Read the model definition and answer for the solid it produces. Units are mm, in the model's axes. Coordinates: 2 decimals unless noted, no trailing zeros.
(1) Straight lines are drawn through the part: line 1 along X through (y, z) = (291.5, -4.5); line 2 along Z through (x, y) = (8.5, 274.5); line 3 along Z through (x, y) = (-12, 164.5). For each, find the intervals that lie inside material, in ascending order.
(2) The part is cut by section A-A, the plane y = 192. State how many separate pieces and enclosed holes the cut face has, and give its area (3 significant figures).
(3) Given pin 1 (1.2 mm diameter, centred on x = -25, y = 241.5, fed in from +Z); pin 2 (0.6 mm diameter, centred on y = 140.5, z = 14.5, fed in from -X); pin 3 (1.3 mm diameter, centred on y = 270, z = 28.5, fed in from +X), each flat-ended and moving along its own axis, determine where each tip first touches the part or whether it passes through.
```python
from build123d import *

# Parameters (mm, degrees)
BOSS_EXTRUDE1_DEPTH = 500


with BuildPart() as part:
    # Sketch1 → Boss-Extrude1 (new body)
    with BuildSketch(Plane(origin=(0, 0, 0), x_dir=(1, 0, 0), z_dir=(0, 1, 0))):
        with BuildLine():
            Line((-27.932618907, -6.859852703), (-27.932618907, 5.140147297))
            ThreePointArc((-27.932618907, 5.140147297), (-26.761046031, 7.968574422), (-23.932618907, 9.140147297))
            Line((-23.932618907, 9.140147297), (-11.932618907, 9.140147297))
            Line((-11.932618907, 9.140147297), (-11.932618907, 4.640147297))
            Line((-11.932618907, 4.640147297), (-19.182618907, 4.640147297))
            Line((-19.182618907, 4.640147297), (-19.182618907, 3.140147297))
            Line((-19.182618907, 3.140147297), (-12.932618907, -3.109852703))
            Line((-12.932618907, -3.109852703), (-7.932618907, -3.109852703))
            Line((-7.932618907, -3.109852703), (-2.932618907, -3.109852703))
            Line((-2.932618907, -3.109852703), (3.317381093, 3.140147297))
            Line((3.317381093, 3.140147297), (3.317381093, 4.640147297))
            Line((3.317381093, 4.640147297), (-3.932618907, 4.640147297))
            Line((-3.932618907, 4.640147297), (-3.932618907, 9.140147297))
            Line((-3.932618907, 9.140147297), (8.067381093, 9.140147297))
            ThreePointArc((8.067381093, 9.140147297), (10.895808218, 7.968574422), (12.067381093, 5.140147297))
            Line((12.067381093, 5.140147297), (12.067381093, -6.859852703))
            Line((12.067381093, -6.859852703), (7.567381093, -6.859852703))
            Line((7.567381093, -6.859852703), (7.567381093, 0.390147297))
            Line((7.567381093, 0.390147297), (6.067381093, 0.390147297))
            Line((6.067381093, 0.390147297), (-0.182618907, -5.859852703))
            Line((-0.182618907, -5.859852703), (-0.182618907, -10.859852703))
            Line((-0.182618907, -10.859852703), (-0.182618907, -15.859852703))
            Line((-0.182618907, -15.859852703), (6.067381093, -22.109852703))
            Line((6.067381093, -22.109852703), (7.567381093, -22.109852703))
            Line((7.567381093, -22.109852703), (7.567381093, -14.859852703))
            Line((7.567381093, -14.859852703), (12.067381093, -14.859852703))
            Line((12.067381093, -14.859852703), (12.067381093, -26.859852703))
            ThreePointArc((12.067381093, -26.859852703), (10.895808218, -29.688279827), (8.067381093, -30.859852703))
            Line((8.067381093, -30.859852703), (-3.932618907, -30.859852703))
            Line((-3.932618907, -30.859852703), (-3.932618907, -26.359852703))
            Line((-3.932618907, -26.359852703), (3.317381093, -26.359852703))
            Line((3.317381093, -26.359852703), (3.317381093, -24.859852703))
            Line((3.317381093, -24.859852703), (-2.932618907, -18.609852703))
            Line((-2.932618907, -18.609852703), (-7.932618907, -18.609852703))
            Line((-7.932618907, -18.609852703), (-12.932618907, -18.609852703))
            Line((-12.932618907, -18.609852703), (-19.182618907, -24.859852703))
            Line((-19.182618907, -24.859852703), (-19.182618907, -26.359852703))
            Line((-19.182618907, -26.359852703), (-11.932618907, -26.359852703))
            Line((-11.932618907, -26.359852703), (-11.932618907, -30.859852703))
            Line((-11.932618907, -30.859852703), (-23.932618907, -30.859852703))
            ThreePointArc((-23.932618907, -30.859852703), (-26.761046031, -29.688279827), (-27.932618907, -26.859852703))
            Line((-27.932618907, -26.859852703), (-27.932618907, -14.859852703))
            Line((-27.932618907, -14.859852703), (-23.432618907, -14.859852703))
            Line((-23.432618907, -14.859852703), (-23.432618907, -22.109852703))
            Line((-23.432618907, -22.109852703), (-21.932618907, -22.109852703))
            Line((-21.932618907, -22.109852703), (-15.682618907, -15.859852703))
            Line((-15.682618907, -15.859852703), (-15.682618907, -10.859852703))
            Line((-15.682618907, -10.859852703), (-15.682618907, -5.859852703))
            Line((-15.682618907, -5.859852703), (-21.932618907, 0.390147297))
            Line((-21.932618907, 0.390147297), (-23.432618907, 0.390147297))
            Line((-23.432618907, 0.390147297), (-23.432618907, -6.859852703))
            Line((-23.432618907, -6.859852703), (-27.932618907, -6.859852703))
        make_face()
        with BuildLine():
            Line((-25.932618907, 2.390147297), (-25.932618907, 5.140147297))
            ThreePointArc((-25.932618907, 5.140147297), (-25.346832469, 6.55436086), (-23.932618907, 7.140147297))
            Line((-23.932618907, 7.140147297), (-21.182618907, 7.140147297))
            Line((-21.182618907, 7.140147297), (-21.182618907, 3.097254079))
            Line((-21.182618907, 3.097254079), (-20.734395602, 2.649030774))
            Line((-20.734395602, 2.649030774), (-21.441502383, 1.941923993))
            Line((-21.441502383, 1.941923993), (-21.889725688, 2.390147297))
            Line((-21.889725688, 2.390147297), (-25.932618907, 2.390147297))
        make_face(mode=Mode.SUBTRACT)
        with BuildLine():
            Line((-20.380842211, 0.881263821), (-13.682618907, -5.816959484))
            Line((-13.682618907, -5.816959484), (-13.682618907, -7.955115193))
            Line((-13.682618907, -7.955115193), (-13.182618907, -7.955115193))
            Line((-13.182618907, -7.955115193), (-12.002324056, -7.955115193))
            ThreePointArc((-12.002324056, -7.955115193), (-11.468152813, -7.324318797), (-10.837356416, -6.790147554))
            Line((-10.837356416, -6.790147554), (-10.837356416, -5.609852703))
            Line((-10.837356416, -5.609852703), (-10.837356416, -5.109852703))
            Line((-10.837356416, -5.109852703), (-12.975512126, -5.109852703))
            Line((-12.975512126, -5.109852703), (-19.67373543, 1.588370602))
            Line((-19.67373543, 1.588370602), (-20.380842211, 0.881263821))
        make_face(mode=Mode.SUBTRACT)
        with BuildLine():
            Line((10.067381093, 2.390147297), (10.067381093, 5.140147297))
            ThreePointArc((10.067381093, 5.140147297), (9.481594656, 6.55436086), (8.067381093, 7.140147297))
            Line((8.067381093, 7.140147297), (5.317381093, 7.140147297))
            Line((5.317381093, 7.140147297), (5.317381093, 3.097254079))
            Line((5.317381093, 3.097254079), (4.869157789, 2.649030774))
            Line((4.869157789, 2.649030774), (5.57626457, 1.941923993))
            Line((5.57626457, 1.941923993), (6.024487874, 2.390147297))
            Line((6.024487874, 2.390147297), (10.067381093, 2.390147297))
        make_face(mode=Mode.SUBTRACT)
        with BuildLine():
            Line((-2.182618907, -5.816959484), (-2.182618907, -7.955115193))
            Line((-2.182618907, -7.955115193), (-2.682618907, -7.955115193))
            Line((-2.682618907, -7.955115193), (-3.862913758, -7.955115193))
            ThreePointArc((-3.862913758, -7.955115193), (-4.397085001, -7.324318797), (-5.027881397, -6.790147554))
            Line((-5.027881397, -6.790147554), (-5.027881397, -5.609852703))
            Line((-5.027881397, -5.609852703), (-5.027881397, -5.109852703))
            Line((-5.027881397, -5.109852703), (-2.889725688, -5.109852703))
            Line((-2.889725688, -5.109852703), (3.808497617, 1.588370602))
            Line((3.808497617, 1.588370602), (4.515604398, 0.881263821))
            Line((4.515604398, 0.881263821), (-2.182618907, -5.816959484))
        make_face(mode=Mode.SUBTRACT)
        with BuildLine():
            Line((5.317381093, -28.859852703), (8.067381093, -28.859852703))
            ThreePointArc((8.067381093, -28.859852703), (9.481594656, -28.274066265), (10.067381093, -26.859852703))
            Line((10.067381093, -26.859852703), (10.067381093, -24.109852703))
            Line((10.067381093, -24.109852703), (6.024487874, -24.109852703))
            Line((6.024487874, -24.109852703), (5.57626457, -23.661629398))
            Line((5.57626457, -23.661629398), (4.869157789, -24.368736179))
            Line((4.869157789, -24.368736179), (5.317381093, -24.816959484))
            Line((5.317381093, -24.816959484), (5.317381093, -28.859852703))
        make_face(mode=Mode.SUBTRACT)
        with BuildLine():
            Line((-2.889725688, -16.609852703), (-5.027881397, -16.609852703))
            Line((-5.027881397, -16.609852703), (-5.027881397, -16.109852703))
            Line((-5.027881397, -16.109852703), (-5.027881397, -14.929557852))
            ThreePointArc((-5.027881397, -14.929557852), (-4.397085001, -14.395386609), (-3.862913758, -13.764590212))
            Line((-3.862913758, -13.764590212), (-2.682618907, -13.764590212))
            Line((-2.682618907, -13.764590212), (-2.182618907, -13.764590212))
            Line((-2.182618907, -13.764590212), (-2.182618907, -15.902745921))
            Line((-2.182618907, -15.902745921), (4.515604398, -22.600969226))
            Line((4.515604398, -22.600969226), (3.808497617, -23.308076007))
            Line((3.808497617, -23.308076007), (-2.889725688, -16.609852703))
        make_face(mode=Mode.SUBTRACT)
        with BuildLine():
            Line((-25.932618907, -24.109852703), (-25.932618907, -26.859852703))
            ThreePointArc((-25.932618907, -26.859852703), (-25.346832469, -28.274066265), (-23.932618907, -28.859852703))
            Line((-23.932618907, -28.859852703), (-21.182618907, -28.859852703))
            Line((-21.182618907, -28.859852703), (-21.182618907, -24.816959484))
            Line((-21.182618907, -24.816959484), (-20.734395602, -24.368736179))
            Line((-20.734395602, -24.368736179), (-21.441502383, -23.661629398))
            Line((-21.441502383, -23.661629398), (-21.889725688, -24.109852703))
            Line((-21.889725688, -24.109852703), (-25.932618907, -24.109852703))
        make_face(mode=Mode.SUBTRACT)
        with BuildLine():
            Line((-13.682618907, -15.902745921), (-13.682618907, -13.764590212))
            Line((-13.682618907, -13.764590212), (-13.182618907, -13.764590212))
            Line((-13.182618907, -13.764590212), (-12.002324056, -13.764590212))
            ThreePointArc((-12.002324056, -13.764590212), (-11.468152813, -14.395386609), (-10.837356416, -14.929557852))
            Line((-10.837356416, -14.929557852), (-10.837356416, -16.109852703))
            Line((-10.837356416, -16.109852703), (-10.837356416, -16.609852703))
            Line((-10.837356416, -16.609852703), (-12.975512126, -16.609852703))
            Line((-12.975512126, -16.609852703), (-19.67373543, -23.308076007))
            Line((-19.67373543, -23.308076007), (-20.380842211, -22.600969226))
            Line((-20.380842211, -22.600969226), (-13.682618907, -15.902745921))
        make_face(mode=Mode.SUBTRACT)
        with BuildLine():
            ThreePointArc((-11.332618907, -10.859852703), (-10.336781963, -8.455689647), (-7.932618907, -7.459852703))
            ThreePointArc((-7.932618907, -7.459852703), (-5.528455851, -8.455689647), (-4.532618907, -10.859852703))
            ThreePointArc((-4.532618907, -10.859852703), (-5.528455851, -13.264015759), (-7.932618907, -14.259852703))
            ThreePointArc((-7.932618907, -14.259852703), (-10.336781963, -13.264015759), (-11.332618907, -10.859852703))
        make_face(mode=Mode.SUBTRACT)
    extrude(amount=BOSS_EXTRUDE1_DEPTH)


solid = part.part
```
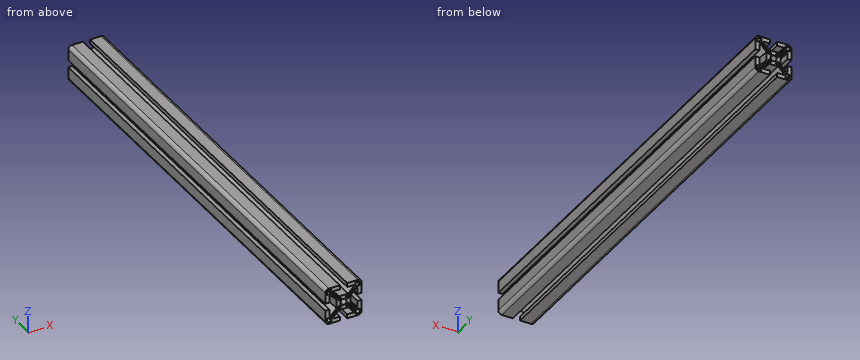
Computed:
1. line 1: x = -27.93 to -25.93, -21.18 to -19.18, 3.32 to 5.32, 10.07 to 12.07
1. line 2: z = -9.12 to -7.09, -2.39 to 6.86, 14.86 to 24.11, 28.81 to 30.84
1. line 3: z = -9.14 to -4.64, 3.11 to 5.11, 7.95 to 13.77, 16.61 to 18.61, 26.36 to 30.86
2. separate pieces: 1
2. enclosed holes: 9
2. area: 710 mm2
3. pin 1: stops at z = 30.83
3. pin 2: stops at x = -15.68
3. pin 3: stops at x = 11.94
